from build123d import *

# Parameters (mm, degrees)
SKETCH1_R           = 1.5
BOSS_EXTRUDE1_DEPTH = 1.25
FILLET2_R           = 10


with BuildPart() as part:
    # Sketch1 → Boss-Extrude1 (new, symmetric)
    with BuildSketch(Plane(origin=(0, 0, 0), x_dir=(1, 0, 0), z_dir=(0, 1, 0))):
        with BuildLine():
            Line((-18.535533906, -11.464466094), (-21.607428337, 0))
            Line((-21.607428337, 0), (-21.607428337, 40))
            Line((-21.607428337, 40), (-18.535533906, 51.464466094))
            Line((-18.535533906, 51.464466094), (-4.393398282, 51.464466094))
            Line((-4.393398282, 51.464466094), (-7.465292714, 40))
            Line((-7.465292714, 40), (-8.465292714, 37.5))
            Line((-8.465292714, 37.5), (-7.465292714, 37.5))
            Line((-7.465292714, 37.5), (-8.465292714, 35))
            Line((-8.465292714, 35), (-7.465292714, 35))
            Line((-7.465292714, 35), (-8.465292714, 32.5))
            Line((-8.465292714, 32.5), (-7.465292714, 32.5))
            Line((-7.465292714, 32.5), (-8.465292714, 30))
            Line((-8.465292714, 30), (-7.465292714, 30))
            Line((-7.465292714, 30), (-8.465292714, 27.5))
            Line((-8.465292714, 27.5), (-7.465292714, 27.5))
            Line((-7.465292714, 27.5), (-8.465292714, 25))
            Line((-8.465292714, 25), (-7.465292714, 25))
            Line((-7.465292714, 25), (-8.465292714, 22.5))
            Line((-8.465292714, 22.5), (-7.465292714, 22.5))
            Line((-7.465292714, 22.5), (-8.465292714, 20))
            Line((-8.465292714, 20), (-7.465292714, 17.5))
            Line((-7.465292714, 17.5), (-8.465292714, 17.5))
            Line((-8.465292714, 17.5), (-7.465292714, 15))
            Line((-7.465292714, 15), (-8.465292714, 15))
            Line((-8.465292714, 15), (-7.465292714, 12.5))
            Line((-7.465292714, 12.5), (-8.465292714, 12.5))
            Line((-8.465292714, 12.5), (-7.465292714, 10))
            Line((-7.465292714, 10), (-8.465292714, 10))
            Line((-8.465292714, 10), (-7.465292714, 7.5))
            Line((-7.465292714, 7.5), (-8.465292714, 7.5))
            Line((-8.465292714, 7.5), (-7.465292714, 5))
            Line((-7.465292714, 5), (-8.465292714, 5))
            Line((-8.465292714, 5), (-7.465292714, 2.5))
            Line((-7.465292714, 2.5), (-8.465292714, 2.5))
            Line((-8.465292714, 2.5), (-7.465292714, 0))
            Line((-7.465292714, 0), (-4.393398282, -11.464466094))
            Line((-4.393398282, -11.464466094), (-39.748737342, -46.819805153))
            ThreePointArc((-39.748737342, -46.819805153), (-46.819805153, -46.819805153), (-46.819805153, -39.748737342))
            Line((-46.819805153, -39.748737342), (-18.535533906, -11.464466094))
        make_face()
        with Locations(Location((-43.284271247, -43.284271247, 0), (0, 0, 270))):
            Circle(SKETCH1_R, mode=Mode.SUBTRACT)
        with Locations(Location((-25.606601718, -25.606601718, 0), (0, 0, 270))):
            Circle(SKETCH1_R, mode=Mode.SUBTRACT)
        with Locations(Location((-15.832428337, 10, 0), (0, 0, 270))):
            Circle(SKETCH1_R, mode=Mode.SUBTRACT)
        with Locations(Location((-13.241481122, -5.732233047, 0), (0, 0, 270))):
            Circle(SKETCH1_R, mode=Mode.SUBTRACT)
        with Locations(Location((-15.832428337, 30, 0), (0, 0, 270))):
            Circle(SKETCH1_R, mode=Mode.SUBTRACT)
        with Locations(Location((-13.241481122, 45.732233047, 0), (0, 0, 270))):
            Circle(SKETCH1_R, mode=Mode.SUBTRACT)
    extrude(amount=BOSS_EXTRUDE1_DEPTH, both=True)

    # Fillet2
    fillet2_edges = [part.edges().sort_by_distance(p)[0] for p in [
        (-21.607428337, 0, 0),
        (-21.607428337, 0, -40),
        (-18.535533906, 0, -51.464466094),
        (-18.535533906, 0, 11.464466094),
    ]]
    fillet(fillet2_edges, radius=FILLET2_R)


solid = part.part
The listing builds one solid part. Answer for the finished solid, in the listing's coordinates (mm). A direction names the side the tool comes from. Coordinates: 2 decimals unless noted, no trailing zeros. Write each loop counter-clockwise with the first axis right and the second up, starting at its lowest first coordinate (ties: lowest second). Pieces come first, ordered by that corner, then holes. Notation, with made-up numbers: (-17.75, -28.5) -> (26.25, -28.5) arc R17 cw to (26.25, 2.5) -> close; hole circle Ø11 at (-12.75, -1.5). An arc over 180 degrees is marked (long way). One line per question, with ' | ' between items.
1. For a pull along X with two mould halves and no side action, classify faces 1 (the flat face through (-21.607, 0, -20)), 2 (the flat face through (-7.972, 0.018, -6.268)), 3 (the cylindrical face through (-17.297, -0.018, -10.325)) as released by +X, released by -X, zero draft, split by the parting line, or undercut.
Verdict:
face 1: released by -X | face 2: released by +X | face 3: undercut
2. Straight lines are drawn through the part: line 1 (Z direction, x = -17, y = 1); line 2 (Z direction, x = -42.5, y = -0.1); line 3 (Z direction, x = -30, y = -0.1). For each, find the intervals that lie inside material, in ascending order.
Verdict:
line 1: z = -49.36 to -30.94, -29.06 to -10.94, -9.06 to 24.07 | line 2: z = 35.43 to 42.01, 44.56 to 48.22 | line 3: z = 22.93 to 37.07
3. Section B-B (x = -29) is taken. Determine the outline of the cut face in (y, z).
Verdict:
outline: (-1.25, 21.93) -> (1.25, 21.93) -> (1.25, 36.07) -> (-1.25, 36.07) -> close
4. Section C-C (z = 13.5) is taken. Determine the outline of the cut face in (x, y), and give its area (3 significant figures).
Verdict:
outline: (-21.04, -1.25) -> (-6.43, -1.25) -> (-6.43, 1.25) -> (-21.04, 1.25) -> close | area: 36.5 mm^2
5. Which of the six approach directions +Z, -Z, +X, -X, +Y, -Y give full straight-line access (tool end or side, diameter ignored) to faces 4 (the flat face through (-7.958, 0.018, -26.268)), 5 (the cylindrical face through (-21.52, -0.02, 0.01)), 6 (the flat face through (-20.9, 0.02, -42.64))?
Verdict:
face 4: +X, +Y, -Y | face 5: -X, +Y, -Y | face 6: -Z, -X, +Y, -Y
6. Given pin 1 Ø1.5 at (y, z) = (-0.5, -21.5) entering from -X; pin 2 Ø0.5 at (x, y) = (-8, 0) entering from +Z; pin 3 Ø5 at (x, z) = (-13.24, -45.73) entering from +Y; pin 4 Ø0.8 at (x, y) = (-8, -0.5) entering from +Z, each flat-ended and moving along its own axis, determine where each tip first touches the part or whether it passes through.
Verdict:
pin 1: stops at x = -21.61 | pin 2: stops at z = 15.32 | pin 3: stops at y = 1.25 | pin 4: stops at z = 15.47
7. Section A-A (y = 0.7) is taken. State how many separate pieces and enclosed holes the cut face has, and give its area (3 significant figures).
Verdict:
separate pieces: 1 | enclosed holes: 6 | area: 1,310 mm^2
